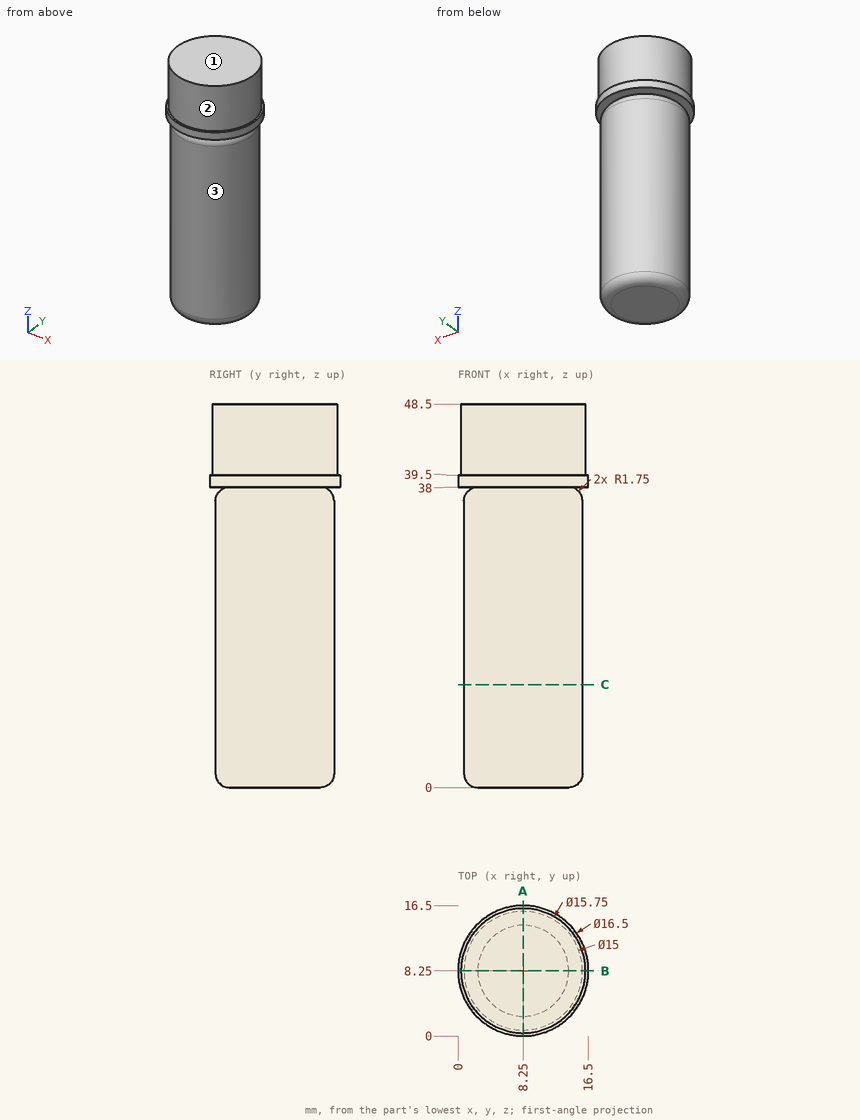
Here's the drawing with two shaded views (mm, measured from the low corner). I have some questions. A direction names the side the tool comes from. Give positions to 0.01 mm unless a question says otherwise; leave off trailing zeros. Write each loop counter-clockwise with the first axis right and the second up, starting at its lowest first coordinate (ties: lowest second). Pieces come first, ordered by that corner, then holes. Notation, with made-up numbers: (-1, -3.75) -> (6, -3.75) arc R32 cw to (6, 30.25) -> close; hole circle Ø9 at (33, 73.5). An arc over 180 degrees is marked (long way). Use one line per item in the form item = value. Start each with the question number.
1. On a 3-axis mill with a long thin cutter (end or side, diameter ignored), from which of +Z, -Z, +X, -X, +Y, -Y can I reach the whole of each face in a straight line? I mean the marked faces 1, 2 and 3. Say none if no direction works.
2. Imagine slicing it at C-C on z = 13. List the corners of the cut face in (x, y) for me.
3. Will these pins go through, and if not, where does the flat tip stop? pin 1 Ø6 at (x, z) = (11.5, 9) entering from +Y; pin 2 Ø4 at (y, z) = (13, 17.5) entering from -X.
4. If I drill on L1, parallel to Z at x = 12.5, y = 1.25; L2, parallel to Z at x = 12.25, y = 2.25; L3, parallel to Z at x = 5.75, y = 1.75, over which ranges is the centre line in solid material (lowest first)?
5. Imagine slicing it at A-A on x = 8.25. List the corners of the cut face in (y, z) for me (3 decimals).
Entries:
q1.face_1 = +Z, +X, -X, +Y, -Y
q1.face_2 = +Z
q1.face_3 = -Z
q2.outline = circle Ø15 at (8.25, 8.25)
q3.pin_1 = 15.75
q3.pin_2 = 1.27
q4.L1 = 38 to 39.5
q4.L2 = 0.79 to 37.21, 38 to 48.5
q4.L3 = 0.49 to 37.51, 38 to 48.5
q5.outline = (0, 38) -> (2.5, 38) arc R1.75 ccw to (0.75, 36.25) -> (0.75, 1.75) arc R1.75 ccw to (2.5, 0) -> (14, 0) arc R1.75 ccw to (15.75, 1.75) -> (15.75, 36.25) arc R1.75 ccw to (14, 38) -> (16.5, 38) -> (16.5, 39.5) -> (16.125, 39.5) -> (16.125, 48.5) -> (0.375, 48.5) -> (0.375, 39.5) -> (0, 39.5) -> close
